Could you check a few things on this model? Use its own coordinates, in mm. Face numbers are marked on the shaded views. A direction names the side the tool comes from. Round coordinates to 2 decimals unless told otherwise and drop trailing zeros. Order: outer loops, then holes, each group sorted by start corner. A loop starts at its lowest first (then second) coordinate and runs counter-clockwise, first axis right, second up. Notation, with made-up numbers: M 10.5,33 L 32.5,33 A17 ccw 32.5,66 Z; hole C -28.5,-12.75 d5. An arc over 180 degrees is marked long. Write each question's results on one line, items separated by ' | '. Start each with the question number.
1. For the marked faces 1, 2 and 3, which set-ups out of +Z, -Z, +X, -X, +Y, -Y let a thin tool reach every point of the face, with its end or its side?
2. Suppose I cut it at B-B on y = -9.25. Write out the boundary of the cut face in (x, z) (3 decimals).
3. We'd pull the mould along Y, two halves only. Please class the marked faces 4, 5 and 6: released by +Y, released by -Y, zero draft, split by the parting line, or undercut.
4. Suppose I cut it at D-D on y = -1. Write out the boundary of the cut face in (x, z), and give its area (3 significant figures).
5. Suppose I cut it at C-C on z = 3.5. Write out the boundary of the cut face in (x, y).
6. Please list where these lines run through material, in increasing order: L1, parallel to Y at x = 3.5, z = 1.25; L2, parallel to X at y = -5.5, z = 1.25; L3, parallel to X at y = 1.75, z = 3.25.
7. I'm going to push flat-ended pins straight in: pin 1 (1.5 mm diameter, centred on y = 6, z = 5, fed in from +X); pin 2 (1.9 mm diameter, centred on y = -2.5, z = 2, fed in from +X); pin 3 (3 mm diameter, centred on x = 5.5, z = 3.5, fed in from +Y). Where does each tip first touch, or does it pass through?
8. Suppose I cut it at A-A on x = 4.75. Write out the boundary of the cut face in (y, z).
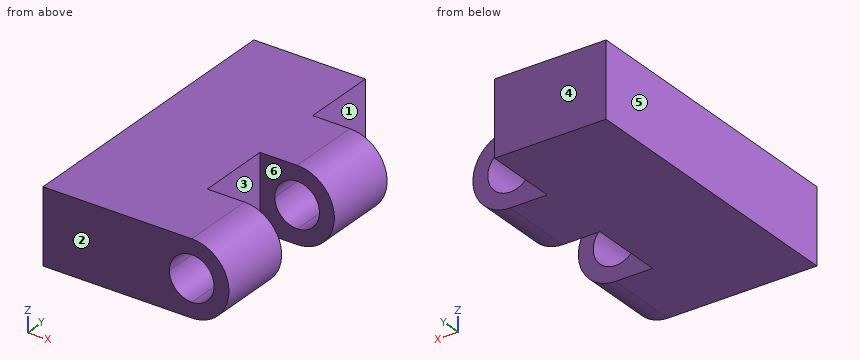
from build123d import *

# Parameters (mm, degrees)
F0_W     = 12.7
F0_H     = 25.4
F1_DEPTH = 6.35
F2_R     = 3.175
F2_R_2   = 1.905
F3_DEPTH = 25.4
F4_DEPTH = 25.4
F5_W     = 6.35
F5_H     = 6.35
F6_DEPTH = 25.4


with BuildPart() as f1:
    # F0 (on Top) → F1 (new body)
    with BuildSketch(Plane.XY):
        Rectangle(F0_W, F0_H)
    extrude(amount=F1_DEPTH)

    # F2 (on face) → F3 (join)
    with BuildSketch(Plane(origin=(0, 12.7, 0), x_dir=(-1, 0, 0), z_dir=(0, 1, 0))):
        with Locations((-6.35, 3.175)):
            Circle(F2_R)
        with Locations((-6.35, 3.175)):
            Circle(F2_R_2, mode=Mode.SUBTRACT)
        with BuildLine():
            ThreePointArc((-4.445, 3.175), (-5.0029615818, 4.5220384182), (-6.35, 5.08))
            Line((-6.35, 5.08), (-6.35, 1.27))
            ThreePointArc((-6.35, 1.27), (-5.0029615818, 1.8279615818), (-4.445, 3.175))
        make_face()
    extrude(amount=-F3_DEPTH)

    # F2 (on face) → F4 (cut)
    with BuildSketch(Plane(origin=(0, 12.7, 0), x_dir=(-1, 0, 0), z_dir=(0, 1, 0))):
        with BuildLine():
            ThreePointArc((-4.445, 3.175), (-5.0029615818, 4.5220384182), (-6.35, 5.08))
            Line((-6.35, 5.08), (-6.35, 1.27))
            ThreePointArc((-6.35, 1.27), (-5.0029615818, 1.8279615818), (-4.445, 3.175))
        make_face()
        with BuildLine():
            Line((-6.35, 1.27), (-6.35, 5.08))
            ThreePointArc((-6.35, 5.08), (-8.255, 3.175), (-6.35, 1.27))
        make_face()
    extrude(amount=-F4_DEPTH, mode=Mode.SUBTRACT)

    # F5 (on face) → F6 (cut)
    with BuildSketch(Plane(origin=(0, 0, 0), x_dir=(1, 0, 0), z_dir=(0, 0, -1))):
        Polygon((3.1755000025, -6.35), (3.1755000025, -12.7), (9.5244999975, -12.7), (9.5255000025, -12.7), (9.5255000025, -6.35), align=None)
        with Locations((6.3505000025, 3.175)):
            Rectangle(F5_W, F5_H)
    extrude(amount=-F6_DEPTH, mode=Mode.SUBTRACT)


solid = f1.part
Filled sheet:
1) face 1: +Z, -Z, +X, +Y | face 2: +Z, -Z, +X, -X, -Y | face 3: +Z, -Z, +X
2) outline: M -6.35,0 L 6.35,0 A3.175 ccw 6.35,6.35 L -6.35,6.35 Z; hole C 6.35,3.175 d3.81
3) face 4: released by +Y | face 5: zero draft | face 6: undercut
4) outline: M -6.35,0 L 3.18,0 L 3.18,6.35 L -6.35,6.35 Z | area: 60.5 mm^2
5) outline: M -6.35,-12.7 L 4.47,-12.7 L 4.47,-6.35 L 3.18,-6.35 L 3.18,0 L 4.47,0 L 4.47,6.35 L 3.18,6.35 L 3.18,12.7 L -6.35,12.7 Z; M 8.23,-12.7 L 9.51,-12.7 L 9.51,-6.35 L 8.23,-6.35 Z; M 8.23,0 L 9.51,0 L 9.51,6.35 L 8.23,6.35 Z
6) L1: y = -12.7 to -6.35, 0 to 6.35 | L2: x = -6.35 to 3.18 | L3: x = -6.35 to 4.45, 8.25 to 9.52
7) pin 1: stops at x = 9.34 | pin 2: stops at x = 3.18 | pin 3: stops at y = 6.35
8) outline: M -12.7,0 L -6.35,0 L -6.35,2.14 L -12.7,2.14 Z; M -12.7,4.21 L -6.35,4.21 L -6.35,6.35 L -12.7,6.35 Z; M 0,0 L 6.35,0 L 6.35,2.14 L 0,2.14 Z; M 0,4.21 L 6.35,4.21 L 6.35,6.35 L 0,6.35 Z
